from build123d import *

# Parameters (mm, degrees)
F0_W     = 152.4
F0_H     = 152.4
F1_DEPTH = 152.4
F5_DEPTH = 50.8


# Not quite as in the source:
# - the program builds the solid bodies; features that only make, move or delete a surface that nothing else refers to are left out


with BuildPart() as f1:
    # F0 (on Top) → F1 (new body)
    with BuildSketch(Plane.XY):
        Rectangle(F0_W, F0_H)
    extrude(amount=F1_DEPTH)

    # F4 (on face) → F5 (cut)
    with BuildSketch(Plane(origin=(0, 76.2, 0), x_dir=(-1, 0, 0), z_dir=(0, 1, 0))):
        Polygon((-1.9910766715, 26.005651243), (36.5384817123, 45.9516048431), (38.5295583838, 89.2921580002), (1.9910766715, 112.6867575571), (-36.5384817123, 92.740803957), (-38.5295583838, 49.4002507999), align=None)
    extrude(amount=-F5_DEPTH, mode=Mode.SUBTRACT)


solid = f1.part
CAD build for the part. Positions are in the model's coordinates, mm. A direction names the side the tool comes from. Coordinates: 2 decimals unless noted, no trailing zeros. Order: outer loops, then holes, each group sorted by start corner. A loop starts at its lowest first (then second) coordinate and runs counter-clockwise, first axis right, second up.
Item 1: Band-saw the part on A-A on y = 67.5. List the corners of the cut face in (x, z).
Check sheet entries:
outline: (-76.2, 0) - (76.2, 0) - (76.2, 152.4) - (-76.2, 152.4) - close; hole (-38.53, 89.29) - (-36.54, 45.95) - (1.99, 26.01) - (38.53, 49.4) - (36.54, 92.74) - (-1.99, 112.69) - close
Item 2: Band-saw the part on B-B on z = 87. List the corners of the cut face in (x, y).
Check sheet entries:
outline: (-76.2, -76.2) - (76.2, -76.2) - (76.2, 76.2) - (36.8, 76.2) - (36.8, 25.4) - (-38.42, 25.4) - (-38.42, 76.2) - (-76.2, 76.2) - close
Item 3: Band-saw the part on C-C on x = -34. List the corners of the cut face in (y, z), plus the area to 3 significant figures.
Check sheet entries:
outline: (-76.2, 0) - (76.2, 0) - (76.2, 44.64) - (25.4, 44.64) - (25.4, 92.19) - (76.2, 92.19) - (76.2, 152.4) - (-76.2, 152.4) - close
area: 20,800 mm2
Item 4: Two-plate mould, pull along Z, no slides. Class faces 1 (the face through (20.52, 51.16, 37.87)), 2 (the face through (17.004, 51.156, 102.853)), 3 (the face through (-1, -76.2, 75)), 4 (the face through (-1, 1, 0)): +Z half, -Z half, draft (parallel to the pull), parting line (faces both ways), or undercut.
Check sheet entries:
face 1: undercut
face 2: undercut
face 3: draft
face 4: -Z half
Item 5: 3-axis set-ups, long thin cutter, end or side, ignore diameter. For faces 5 (the face through (-18, 76.2, 109)), 6 (the face through (37.52, 51.16, 71.37)): which of +Z, -Z, +X, -X, +Y, -Y reach the whole face in a straight line?
Check sheet entries:
face 5: +Z, -Z, +X, -X, +Y
face 6: +Y
Item 6: Drill centre lines: L1, parallel to Z at x = 27.5, y = 40; L2, parallel to Y at x = -17.5, z = 65; L3, parallel to X at y = 56, z = 88. Where is each one in solid material? Low to high.
Check sheet entries:
L1: z = 0 to 42.34, 97.42 to 152.4
L2: y = -76.2 to 25.4
L3: x = -76.2 to -38.47, 36.76 to 76.2
